Read the model definition and answer for the solid it produces. Units are mm, in the model's axes. Give positions to 0.01 mm unless a question says otherwise; leave off trailing zeros. Write each loop counter-clockwise with the first axis right and the second up, starting at its lowest first coordinate (ties: lowest second). Pieces come first, ordered by that corner, then holes.
```python
from build123d import *

# Parameters (mm, degrees)
SKETCH1_W            = 44.45
SKETCH1_H            = 247.65
BOSS_EXTRUDE1_DEPTH  = 6.35
M4_CLEARANCE_HOLE1_D = 4.8


with BuildPart() as part:
    # Sketch1 → Boss-Extrude1 (new body)
    with BuildSketch(Plane(origin=(0, 0, 0), x_dir=(1, 0, 0), z_dir=(0, 1, 0))):
        Rectangle(SKETCH1_W, SKETCH1_H)
    extrude(amount=BOSS_EXTRUDE1_DEPTH)

    # M4 Clearance Hole1 (through all)
    with Locations(Plane(origin=(0, 0, 0), x_dir=(-1, 0, 0), z_dir=(0, -1, 0))):
        with Locations((37.2, -116.6), (5.2, -116.6), (5.2, -86.6), (37.2, -86.6), (37.2, 86.6), (37.2, 116.6), (5.2, 116.6), (5.2, 86.6)):
            Hole(M4_CLEARANCE_HOLE1_D / 2)


solid = part.part
```
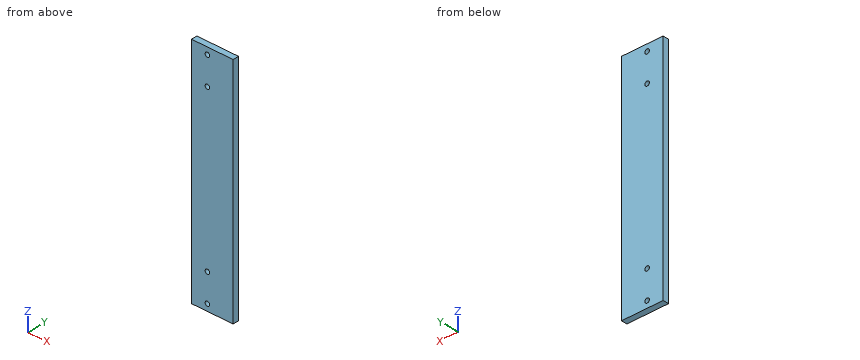
Item 1: Section A-A (z = -116.6) is taken. Write down the section's boundary in (x, y) (3 decimals), and give its area (3 significant figures).
Result set:
outline: (-22.225, 0) - (-7.6, 0) - (-7.6, 6.35) - (-22.225, 6.35) - close; (-2.8, 0) - (22.225, 0) - (22.225, 6.35) - (-2.8, 6.35) - close
area: 252 mm2
Item 2: Find the intervals of material crossed by line 1 along Z through (x, y) = (-5.2, 3) (3 decimals); line 2 along X through (y, z) = (3.25, 86.6) (3 decimals); line 3 along Z through (x, y) = (-4.5, 6) (3 decimals), in increasing order.
Result set:
line 1: z = -123.825 to -119, -114.2 to -89, -84.2 to 84.2, 89 to 114.2, 119 to 123.825
line 2: x = -22.225 to -7.6, -2.8 to 22.225
line 3: z = -123.825 to -118.896, -114.304 to -88.896, -84.304 to 84.304, 88.896 to 114.304, 118.896 to 123.825
Item 3: Section B-B (x = -5.2) is taken. Write down the section's boundary in (y, z) (3 decimals).
Result set:
outline: (0, -123.825) - (6.35, -123.825) - (6.35, -119) - (0, -119) - close; (0, -114.2) - (6.35, -114.2) - (6.35, -89) - (0, -89) - close; (0, -84.2) - (6.35, -84.2) - (6.35, 84.2) - (0, 84.2) - close; (0, 89) - (6.35, 89) - (6.35, 114.2) - (0, 114.2) - close; (0, 119) - (6.35, 119) - (6.35, 123.825) - (0, 123.825) - close
Item 4: This flat-tipped pin is pushed along its axis until it touches: pin 1 Ø4 at (x, z) = (-5.2, -86.6) entering from -Y. Where does it stop, or does it pass through?
Result set:
pin 1: passes through
